Autodesk Inventor part; units mm, degrees
ref_plane "Work Plane2" through (3.666174, 6.35, -16.4719) normal (0, 0, -1) x (-1, 0, 0)
ref_plane "Work Plane3" through (0, 0, -6.4389) normal (0, 0, -1) x (-1, 0, 0)
ref_plane "YZ Plane" through (0, 0, 0) normal (1, 0, 0) x (0, 1, 0)
sketch "Sketch1" plane through (0, 0, 0) normal (0, 0, 1) x (1, 0, 0)
  line L0 (-3.666174, 6.35) -> (3.666174, 6.35)
  line L1 (3.666174, 6.35) -> (7.332348, 0)
  line L2 (7.332348, 0) -> (3.666174, -6.35)
  line L3 (3.666174, -6.35) -> (-3.666174, -6.35)
  line L4 (-3.666174, -6.35) -> (-7.332348, 0)
  line L5 (-7.332348, 0) -> (-3.666174, 6.35)
  line L6 (-10.265288, 0) -> (10.265288, 0)
  line L7 (0, -8.89) -> (0, 8.89)
  point P0 (0, 0)
  point P1 (0, 0)
  dimension "d0" = 12.7
extrude "Extrusion1" add sketch "Sketch1" along normal mid plane 78.5622
sketch "Sketch5" plane through (0, 0, 39.2811) normal (0, 0, 1) x (1, 0, 0)
  line L0 (3.666174, 6.35) -> (7.332348, 0)
  line L1 (-3.666174, 6.35) -> (3.666174, 6.35)
  line L2 (-7.332348, 0) -> (-3.666174, 6.35)
  line L3 (-3.666174, -6.35) -> (-7.332348, 0)
  line L4 (3.666174, -6.35) -> (-3.666174, -6.35)
  line L5 (7.332348, 0) -> (3.666174, -6.35)
  circle A0 centre (0, 0) radius 6.35
extrude "Bearing Insert" cut sketch "Sketch5" against normal blind 7.9502 contours L0 A0 L1 | L0 L5 A0 | A0 L2 L1 | A0 L3 L2 | L5 L4 A0 | A0 L4 L3
mirror "Bearing Insert Mirror" about plane through (0, 0, 0) normal (0, 0, 1) of "Bearing Insert"
sketch "Sketch6" plane through (0, 0, -39.2811) normal (0, 0, -1) x (-1, 0, 0)
  circle A0 centre (0, 0) radius 6.35
  circle A1 centre (0, 0) radius 3.175
  dimension "d11" = 6.35
extrude "Extrusion5" cut sketch "Sketch6" against normal blind 15.875 contours A1
ref_plane "Work Plane2" through (3.666174, 6.35, -16.4719) normal (0, 0, -1) x (-1, 0, 0)
sketch "Sketch7" plane through (3.666174, 6.35, -16.4719) normal (0, 0, -1) x (-1, 0, 0)
  line L0 (0, 0) -> (3.666174, 0)
  line L1 (-1.833087, -3.175) -> (0, 0)
  circle A0 centre (3.666174, -6.35) radius 5.0292
  circle A1 centre (3.666174, -6.35) radius 7.332348
  dimension "d16" = 10.0584
extrude "Extrusion6" cut sketch "Sketch7" along normal blind 1.1684
ref_plane "Work Plane3" through (0, 0, -6.4389) normal (0, 0, -1) x (-1, 0, 0)
sketch "Sketch8" plane through (0, 0, -6.4389) normal (0, 0, -1) x (-1, 0, 0)
  line L0 (5.499261, 3.175) -> (7.332348, 0)
  line L1 (7.332348, 0) -> (5.499261, -3.175)
  circle A0 centre (0, 0) radius 5.0292
  circle A1 centre (0, 0) radius 7.332348
  point P0 (0, 0)
  dimension "d20" = 10.0584
extrude "Extrusion7" cut sketch "Sketch8" against normal blind 1.1684
sketch "Sketch9" plane through (0, 0, 39.2811) normal (0, 0, 1) x (1, 0, 0)
  circle A0 centre (0, 0) radius 6.35
  line L0 (-3.666174, 6.35) -> (0, 6.35)
  line L1 (-5.499261, 3.175) -> (-3.666174, 6.35)
  circle A1 centre (0, 0) radius 7.332348
sketch "Sketch9 outline for Extrusion8" plane through (0, 0, 39.2811) normal (0, 0, 1) x (1, 0, 0)
  circle A0 centre (0, 0) radius 7.332348
  arc A1 (-5.499261, 3.175) -> (0, 6.35) centre (0, 0) ccw
  arc A2 (0, 6.35) -> (-5.499261, 3.175) centre (0, 0) ccw
extrude "Extrusion8" cut sketch "Sketch9 outline for Extrusion8" against normal blind 19.05
sketch "Sketch10" plane through (0, 0, 39.2811) normal (0, 0, 1) x (1, 0, 0)
  circle A0 centre (0, 0) radius 6.35
  line L0 (-1.5875, 6.148361) -> (-1.5875, 4.560861)
  line L1 (-1.5875, 4.560861) -> (1.5875, 4.560861)
  line L2 (1.5875, 4.560861) -> (1.5875, 6.148361)
  line L3 (-10.265288, 0) -> (10.265288, 0)
  line L4 (0, -8.89) -> (0, 8.89)
  point P0 (0, 4.560861)
  dimension "d25" = 3.175
  dimension "d26" = 1.5875
extrude "Extrusion9" cut sketch "Sketch10" against normal up to surface (19.05 mm away) contours L2 L1 L4 A0 | L4 L1 L0 A0
equation "\"d26\" = 0.5 * d25"
properties part number "output_shaft" material "Steel"
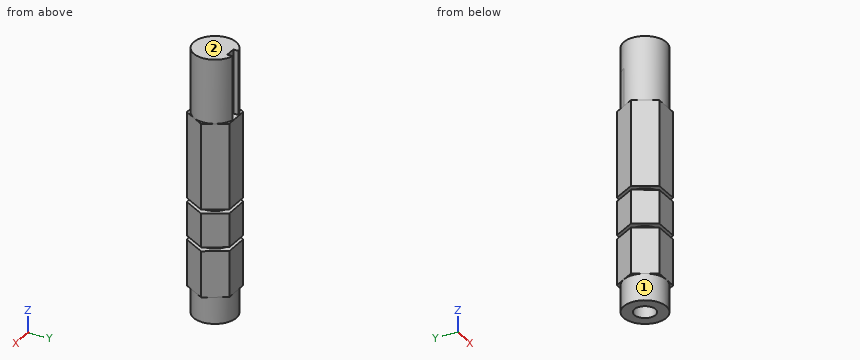
Build history of the part. All positions in model axes, mm. Face numbers are marked on the shaded views. A direction names the side the tool comes from. Coordinates: 2 decimals unless noted, no trailing zeros. Order: outer loops, then holes, each group sorted by start corner. A loop starts at its lowest first (then second) coordinate and runs counter-clockwise, first axis right, second up. Notation, with made-up numbers: (-5.5, 6) - (50.5, 6) arc R23 cw to (50.5, 22) - close; hole circle Ø2 at (44, 22.5). An arc over 180 degrees is marked (long way). Write each question's results on one line, items separated by ' | '. Start each with the question number.
Item 1: Wall check: probe 1 along Z at (x, y) = (5.25, 1); probe 2 along Y at (x, z) = (0, -31.5) (3 decimals); probe 3 along Z at (x, y) = (1, 5.25). Give the ranges that are in metal, low to high. Write a range as [from, to].
Item 2: Flat gauge pins, fed straight in: pin 1 (1.3 mm diameter, centred on y = 5.5, z = 25.5, fed in from -X); pin 2 (3 mm diameter, centred on x = 5.5, z = 1.5, fed in from +Y); pin 3 (2 mm diameter, centred on y = 0.5, z = -9, fed in from +X). Where does each tip first touch, or does it go through?
Item 3: Band-saw the part on A-A on z = 14. Write the cut outline in (x, y), and give its area (3 significant figures).
Item 4: Tool access for the marked faces 1 and 2: list every direction of +Z, -Z, +X, -X, +Y, -Y with a clear straight run to the whole face (end or side of a thin tool).
Numbers:
1) probe 1: [-39.28, -17.64], [-16.47, -6.44], [-5.27, 39.28] | probe 2: [-6.35, -3.175], [3.175, 6.35] | probe 3: [-39.28, -17.64], [-16.47, -6.44], [-5.27, 20.23]
2) pin 1: x = -4.1 | pin 2: y = 5.77 | pin 3: x = 7.33
3) outline: (-7.33, 0) - (-3.67, -6.35) - (3.67, -6.35) - (7.33, 0) - (3.67, 6.35) - (-3.67, 6.35) - close | area: 140 mm^2
4) face 1: -Z | face 2: +Z, +X, -X, +Y, -Y
